Geometry check sheet. Reference: the model listing, model coordinates, mm. Round coordinates to 2 decimals unless told otherwise and drop trailing zeros. Order: outer loops, then holes, each group sorted by start corner. A loop starts at its lowest first (then second) coordinate and runs counter-clockwise, first axis right, second up.
```python
from build123d import *

# Parameters (mm, degrees)
SKETCH1_R           = 2.25
SKETCH1_R_2         = 2.75
BOSS_EXTRUDE1_DEPTH = 7.5


with BuildPart() as part:
    # Sketch1 → Boss-Extrude1 (new body)
    with BuildSketch(Plane(origin=(0, 0, 0), x_dir=(1, 0, 0), z_dir=(0, 1, 0))):
        with BuildLine():
            Line((-166, -10), (76, -10))
            ThreePointArc((76, -10), (78.828427125, -8.828427125), (80, -6))
            Line((80, -6), (80, 44.5))
            Line((80, 44.5), (39.502647377, 117.931699085))
            ThreePointArc((39.502647377, 117.931699085), (38.033863769, 119.444328406), (36, 120))
            Line((36, 120), (-124, 120))
            ThreePointArc((-124, 120), (-156.526911935, 106.526911935), (-170, 74))
            Line((-170, 74), (-170, -6))
            ThreePointArc((-170, -6), (-168.828427125, -8.828427125), (-166, -10))
        make_face()
        with Locations(Location((65, 0, 0), (0, 0, 270))):
            Circle(SKETCH1_R, mode=Mode.SUBTRACT)
        with Locations(Location((-45, 0, 0), (0, 0, 270))):
            Circle(SKETCH1_R, mode=Mode.SUBTRACT)
        with Locations(Location((-155, 0, 0), (0, 0, 270))):
            Circle(SKETCH1_R, mode=Mode.SUBTRACT)
        with Locations(Location((0, 90, 0), (0, 0, 270))):
            Circle(SKETCH1_R_2, mode=Mode.SUBTRACT)
        with Locations(Location((0, 110, 0), (0, 0, 270))):
            Circle(SKETCH1_R_2, mode=Mode.SUBTRACT)
        with Locations(Location((0, 30, 0), (0, 0, 270))):
            Circle(SKETCH1_R, mode=Mode.SUBTRACT)
    extrude(amount=BOSS_EXTRUDE1_DEPTH)


solid = part.part
```
(1) Sectioned sample at B-B, the plane z = -110. Record the cut outline in (x, y), and give its area (3 significant figures).
Returned:
outline: (-152.64, 0) - (-2.75, 0) - (-2.75, 7.5) - (-152.64, 7.5) - close; (2.75, 0) - (43.88, 0) - (43.88, 7.5) - (2.75, 7.5) - close
area: 1,430 mm2
(2) Material ranges on line 1 (X direction, y = 4.5, z = 0); line 2 (X direction, y = 5.5, z = -30); line 3 (X direction, y = 4.5, z = -90), recorded low to high.
Returned:
line 1: x = -170 to -157.25, -152.75 to -47.25, -42.75 to 62.75, 67.25 to 80
line 2: x = -170 to -2.25, 2.25 to 80
line 3: x = -167.13 to -2.75, 2.75 to 54.91
(3) Draft check along Z on faces 1 (the flat face through (-47, 7.5, -56)), 2 (the cylindrical face through (62.804, 3.698, -0.488)), 3 (the flat face through (-47, 4, 10)). Enter one of: released by +Z, released by -Z, zero draft, split by the parting line, or undercut.
Returned:
face 1: zero draft
face 2: undercut
face 3: released by +Z
(4) Sectioned sample at A-A, the plane y = 1.5. Record the cut outline in (x, z).
Returned:
outline: (-170, -74) arc R46 ccw to (-124, -120) - (36, -120) arc R4 ccw to (39.5, -117.93) - (80, -44.5) - (80, 6) arc R4 ccw to (76, 10) - (-166, 10) arc R4 ccw to (-170, 6) - close; hole circle Ø4.5 at (-155, 0); hole circle Ø4.5 at (-45, 0); hole circle Ø5.5 at (0, -110); hole circle Ø5.5 at (0, -90); hole circle Ø4.5 at (0, -30); hole circle Ø4.5 at (65, 0)
(5) Depth check by flat-ended pin: P1, Ø2.5, axis at x = 0, z = -30, coming from the -Y side; P2, Ø3, axis at y = 2.5, z = -83.5, coming from the -X side. Enter the tip coordinate at first touch or a pass-through.
Returned:
P1: passes through
P2: stops at x = -169.3
